Can you work these out from the model? Positions are in its coordinate system, mm. A direction names the side the tool comes from. Round coordinates to 2 decimals unless told otherwise and drop trailing zeros. Order: outer loops, then holes, each group sorted by start corner. A loop starts at its lowest first (then second) coordinate and runs counter-clockwise, first axis right, second up.
Q1. Will these pins go through, and if not, where does the flat tip stop? P1, Ø1.5, axis at x = 44.5, z = -18.5, coming from the -Y side; P2, Ø1.5, axis at y = -18.5, z = -14.5, coming from the +X side.
Q2. If we section it at A-A (x = 42.15): Please give me the cut outline in (y, z), plus the area to 3 significant figures.
Q3. For faces 4 (the face through (10.575, 22.157, 6.734)), 5 (the face through (13, 11, 11.999)), 6 (the face through (1.479, -26.953, 4.817)), which set-ups out of +Z, -Z, +X, -X, +Y, -Y let a thin tool reach every point of the face, with its end or its side?
Q4. We'd pull the mould along Y, two halves only. Please class faces 1 (the face through (1, -4, -23.001)), 2 (the face through (42.6, 22.16, -24.22)), 3 (the face through (1.48, -27.4, 12.46)): pulls with the +Y half, pulls with the -Y half, needs draft (parallel to the pull), parting line crosses it, or undercut.
Q5. If we section it at D-D (x = 26.65): Please give me the cut outline in (y, z), plus the area to 3 significant figures.
Q6. If we section it at C-C (z = -2.5): Please give me the cut outline in (x, y).
Q7. If I drill on line 1 (Z direction, x = 2.5, y = -1); line 2 (Z direction, x = 11, y = 22); line 3 (Z direction, x = 7.5, y = 11.5), over which ranges is the centre line in solid material (lowest first)?
Q8. If we section it at B-B (y = -11): Please give me the cut outline in (x, z), plus the area to 3 significant figures.
from build123d import *

# Parameters (mm, degrees)
SKETCH1_W           = 50.3
SKETCH1_H           = 53.5
BOSS_EXTRUDE1_DEPTH = 3
SKETCH3_W           = 50.3
SKETCH3_H           = 3
BOSS_EXTRUDE3_DEPTH = 50.3
BOSS_EXTRUDE6_DEPTH = 3
BOSS_EXTRUDE7_DEPTH = 3
SKETCH12_R          = 1.5
SKETCH12_R_2        = 11.075
CUT_EXTRUDE1_DEPTH  = 3
CHAMFER2_SIZE       = 5
CHAMFER3_SIZE       = 5
CHAMFER4_SIZE       = 5
CHAMFER5_SIZE       = 5


with BuildPart() as part:
    # Sketch1 → Boss-Extrude1 (new body)
    with BuildSketch(Plane(origin=(0, 0, 0), x_dir=(0, 0, -1), z_dir=(1, 0, 0))):
        with Locations((10.151141702, -3.113798218)):
            Rectangle(SKETCH1_W, SKETCH1_H)
        with BuildLine():
            Line((-6.998858298, -24.818417552), (-6.998858298, 18.3151534))
            ThreePointArc((-6.998858298, 18.3151534), (-4.863858298, 20.4501534), (-2.728858298, 18.3151534))
            Line((-2.728858298, 18.3151534), (-2.728858298, -24.818417552))
            ThreePointArc((-2.728858298, -24.818417552), (-4.863858298, -26.953417552), (-6.998858298, -24.818417552))
        make_face(mode=Mode.SUBTRACT)
        with BuildLine():
            Line((27.271141702, 18.3151534), (27.271141702, -24.818417552))
            ThreePointArc((27.271141702, -24.818417552), (25.136141702, -26.953417552), (23.001141702, -24.818417552))
            Line((23.001141702, -24.818417552), (23.001141702, 18.3151534))
            ThreePointArc((23.001141702, 18.3151534), (25.136141702, 20.4501534), (27.271141702, 18.3151534))
        make_face(mode=Mode.SUBTRACT)
    extrude(amount=BOSS_EXTRUDE1_DEPTH)

    # Sketch3 → Boss-Extrude3 (add)
    with BuildSketch(Plane(origin=(3, 0, 0), x_dir=(0, 0, -1), z_dir=(1, 0, 0))):
        with Locations((10.151141702, 22.136201782)):
            Rectangle(SKETCH3_W, SKETCH3_H)
    extrude(amount=BOSS_EXTRUDE3_DEPTH)

    # Sketch11 → Boss-Extrude6 (add)
    with BuildSketch(Plane.XY.offset(14.998858298)):
        Polygon((3, 20.636201782), (3, -4.613798218), (28.15, 20.636201782), align=None)
    extrude(amount=-BOSS_EXTRUDE6_DEPTH)

    # Sketch7 → Boss-Extrude7 (add)
    with BuildSketch(Plane(origin=(0, 0, -35.301141702), x_dir=(-1, 0, 0), z_dir=(0, 0, -1))):
        Polygon((-3, 20.636201782), (-28.15, 20.636201782), (-3, -3.113798218), align=None)
    extrude(amount=-BOSS_EXTRUDE7_DEPTH)

    # Sketch12 → Cut-Extrude1 (cut)
    with BuildSketch(Plane(origin=(0, 23.636201782, 0), x_dir=(1, 0, 0), z_dir=(0, 1, 0))):
        with Locations(Location((42.15, 25.651141702, 0), (0, 0, 270))):
            Circle(SKETCH12_R)
        with Locations(Location((42.15, -5.348858298, 0), (0, 0, 270))):
            Circle(SKETCH12_R)
        with Locations(Location((11.15, 25.651141702, 0), (0, 0, 270))):
            Circle(SKETCH12_R)
        with Locations(Location((11.15, -5.348858298, 0), (0, 0, 270))):
            Circle(SKETCH12_R)
        with Locations(Location((26.65, 10.151141702, 0), (0, 0, 270))):
            Circle(SKETCH12_R_2)
    extrude(amount=-CUT_EXTRUDE1_DEPTH, mode=Mode.SUBTRACT)

    # Chamfer2
    chamfer2_edges = [part.edges().sort_by_distance(p)[0] for p in [
        (53.3, 22.136201782, -35.301141702),
    ]]
    chamfer(chamfer2_edges, length=CHAMFER2_SIZE)

    # Chamfer3
    chamfer3_edges = [part.edges().sort_by_distance(p)[0] for p in [
        (53.3, 22.136201782, 14.998858298),
    ]]
    chamfer(chamfer3_edges, length=CHAMFER3_SIZE)

    # Chamfer4
    chamfer4_edges = [part.edges().sort_by_distance(p)[0] for p in [
        (1.5, -29.863798218, 14.998858298),
    ]]
    chamfer(chamfer4_edges, length=CHAMFER4_SIZE)

    # Chamfer5
    chamfer5_edges = [part.edges().sort_by_distance(p)[0] for p in [
        (1.5, -29.863798218, -35.301141702),
    ]]
    chamfer(chamfer5_edges, length=CHAMFER5_SIZE)


solid = part.part
Solution:
1. P1: stops at y = 20.64
1. P2: stops at x = 3
2. outline: (20.64, -35.3) - (23.64, -35.3) - (23.64, -27.15) - (20.64, -27.15) - close; (20.64, -24.15) - (23.64, -24.15) - (23.64, 3.85) - (20.64, 3.85) - close; (20.64, 6.85) - (23.64, 6.85) - (23.64, 15) - (20.64, 15) - close
2. area: 133 mm2
3. face 4: +Y, -Y
3. face 5: +X, -Y
3. face 6: +X, -X
4. face 1: undercut
4. face 2: needs draft
4. face 3: pulls with the -Y half
5. outline: (19.13, 12) - (20.64, 12) - (20.64, 0.92) - (23.64, 0.92) - (23.64, 15) - (19.13, 15) - close; (19.22, -35.3) - (23.64, -35.3) - (23.64, -21.23) - (20.64, -21.23) - (20.64, -32.3) - (19.22, -32.3) - close
5. area: 93.2 mm2
6. outline: (0, -29.86) - (3, -29.86) - (3, 20.64) - (18.64, 20.64) - (18.64, 23.64) - (0, 23.64) - close; (34.66, 20.64) - (53.3, 20.64) - (53.3, 23.64) - (34.66, 23.64) - close
7. line 1: z = -35.3 to -27.27, -23 to 2.73, 7 to 15
7. line 2: z = -35.3 to -27.14, -24.16 to 3.86, 6.84 to 15
7. line 3: z = -35.3 to -32.3, 12 to 15
8. outline: (0, -35.3) - (3, -35.3) - (3, -27.27) - (0, -27.27) - close; (0, -23) - (3, -23) - (3, 2.73) - (0, 2.73) - close; (0, 7) - (3, 7) - (3, 15) - (0, 15) - close
8. area: 125 mm2
